Geometry: see drawing. Coordinates: mm, zero at the bounding-box minimum. Coordinates: 2 decimals unless noted, no trailing zeros. Write each loop counter-clockwise with the first axis right and the second up, starting at its lowest first coordinate (ties: lowest second). Pieces come first, ordered by that corner, then holes. Notation, with made-up numbers: (4.5, 74) -> (36.5, 74) arc R27 cw to (36.5, 112) -> close; hole circle Ø9 at (-6.75, 60.5). An arc over 180 degrees is marked (long way). Use one line per item in the form item = value. Start each with the question number.
(1) Cut plane A-A on y = 1.45. Return the cut outline in (x, z).
(2) Ray query, line 1 along X through (y, z) = (0.35, 26); line 2 along Z through (x, y) = (14, 0.35) (1 decimal); line 3 along Z through (x, y) = (20.25, 0.35) (1 decimal). Return the intervals inside material, ascending.
(3) Cut plane C-C on x = 22. Return the cut outline in (y, z).
(4) Cut plane B-B on z = 33.5. Return the cut outline in (x, y).
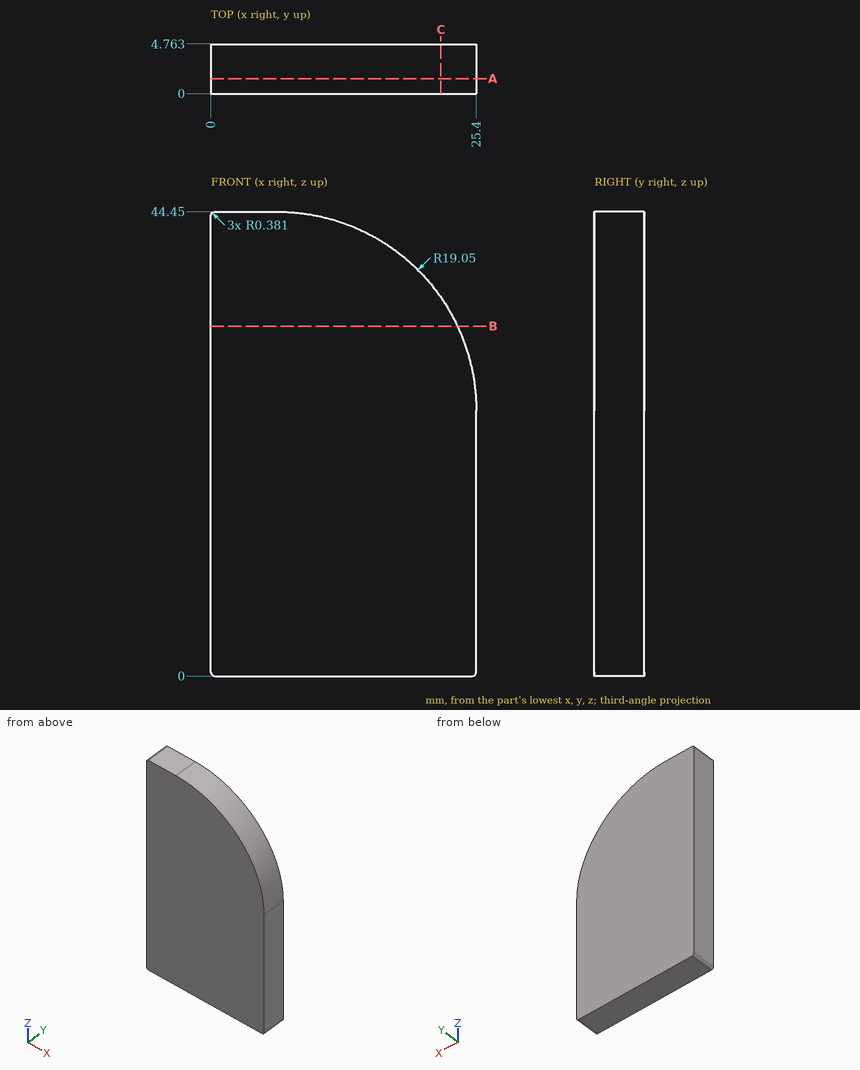
Values:
q1.outline = (0, 0.38) arc R0.38 ccw to (0.38, 0) -> (25.02, 0) arc R0.38 ccw to (25.4, 0.38) -> (25.4, 25.4) arc R19.05 ccw to (6.35, 44.45) -> (0.38, 44.45) arc R0.38 ccw to (0, 44.07) -> close
q2.line_1 = 0 to 25.39
q2.line_2 = 0 to 42.8
q2.line_3 = 0 to 38.4
q3.outline = (0, 0) -> (4.76, 0) -> (4.76, 36.26) -> (0, 36.26) -> close
q4.outline = (0, 0) -> (23.59, 0) -> (23.59, 4.76) -> (0, 4.76) -> close
